Verification items for this drawing (mm, ordinates from the low corner). A direction names the side the tool comes from. Coordinates: 2 decimals unless noted, no trailing zeros. Order: outer loops, then holes, each group sorted by start corner. A loop starts at its lowest first (then second) coordinate and runs counter-clockwise, first axis right, second up. Notation, with made-up numbers: M 72,-21.5 L 97,-21.5 A24 cw 97,13.5 Z; hole C 75,53 d8. An arc over 180 degrees is marked long. Write item = value, one per line.
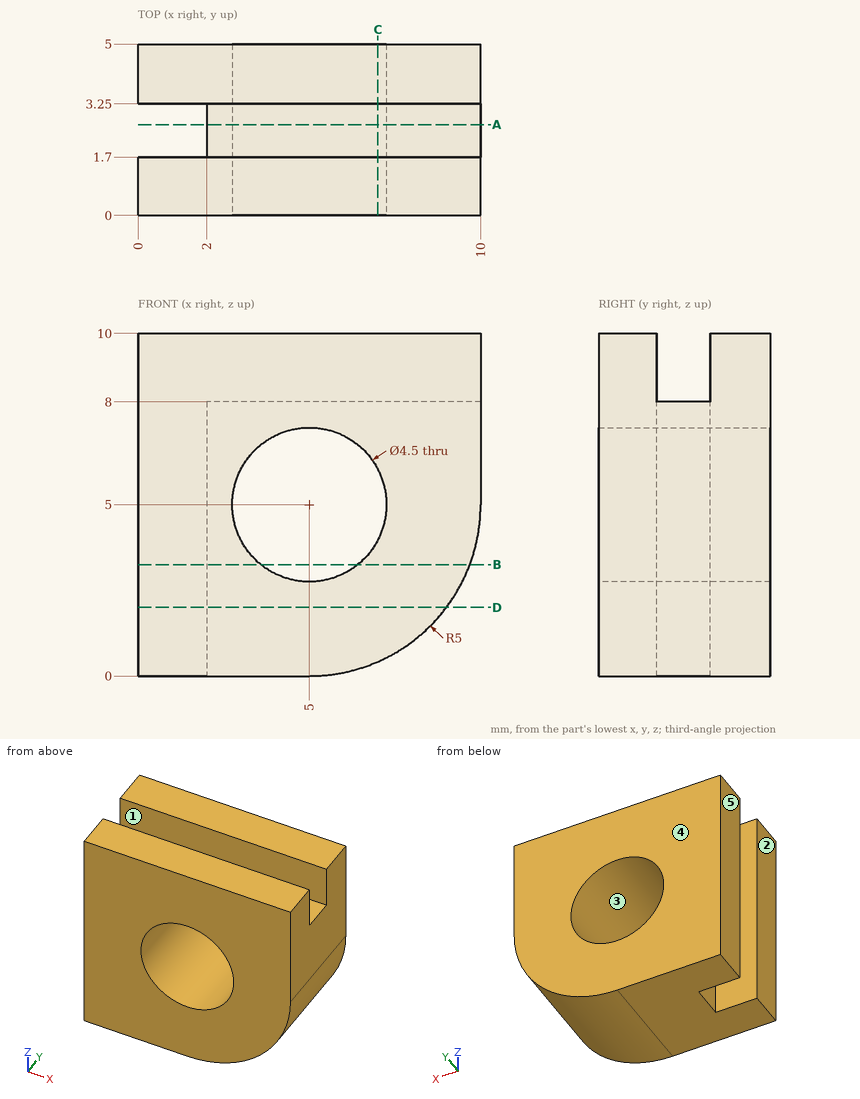
Item 1: Sectioned sample at C-C, the plane x = 7. Enter the section's corners in (y, z).
Report:
outline = M 0,0.42 L 5,0.42 L 5,3.97 L 0,3.97 Z; M 0,6.03 L 5,6.03 L 5,10 L 3.25,10 L 3.25,8 L 1.7,8 L 1.7,10 L 0,10 Z
Item 2: Sectioned sample at B-B, the plane z = 3.25. Enter the section's corners in (x, y).
Report:
outline = M 0,0 L 3.59,0 L 3.59,5 L 0,5 L 0,3.25 L 2,3.25 L 2,1.7 L 0,1.7 Z; M 6.41,0 L 9.68,0 L 9.68,5 L 6.41,5 Z
Item 3: Sectioned sample at D-D, the plane z = 2. Enter the section's corners in (x, y), then the cut area to 3 significant figures.
Report:
outline = M 0,0 L 9,0 L 9,5 L 0,5 L 0,3.25 L 2,3.25 L 2,1.7 L 0,1.7 Z
area = 41.9 mm^2
Item 4: Sectioned sample at A-A, the plane y = 2.65. Enter the section's corners in (x, z), then the cut area to 3 significant figures.
Report:
outline = M 2,0 L 5,0 A5 ccw 10,5 L 10,8 L 2,8 Z; hole C 5,5 d4.5
area = 42.7 mm^2
Item 5: Release check for a two-part mould opening along X. For the marked faces 3, 4 and 5 record: pulls with the +X half, pulls with the -X half, needs draft (parallel to the pull), parting line crosses it, or undercut.
Report:
face_3 = undercut
face_4 = needs draft
face_5 = pulls with the -X half
Item 6: Scan lines: L1, parallel to X at y = 1.35, z = 5; L2, parallel to Y at x = 1.5, z = 2.25; L3, parallel to X at y = 2.9, z = 5. Record each from-to range of solid material in increasing order. Write a range as from..to.
Report:
L1 = 0..2.75, 7.25..10
L2 = 0..1.7, 3.25..5
L3 = 2..2.75, 7.25..10
Item 7: Tool access check on the marked faces 1 and 2. Record the directions out of +Z, -Z, +X, -X, +Y, -Y that give a thin tool (end or side, any length) a straight path to the whole face; none if there is none.
Report:
face_1 = +Z, -X
face_2 = +Z, -Z, -X, +Y, -Y
